Here's how the part is built. I have some questions about the finished solid (model axes, mm). A direction names the side the tool comes from. Coordinates: 2 decimals unless noted, no trailing zeros. Write each loop counter-clockwise with the first axis right and the second up, starting at its lowest first coordinate (ties: lowest second). Pieces come first, ordered by that corner, then holes. Notation, with made-up numbers: (76.5, 18) -> (93.5, 18) arc R14 cw to (93.5, 33) -> close; hole circle Ø2 at (-0.75, 37.5). An arc over 180 degrees is marked (long way). Put each result on its own line as item: value.
```python
from build123d import *

# Parameters (mm, degrees)
SKETCH1_W           = 40
SKETCH1_H           = 40
BOSS_EXTRUDE1_DEPTH = 25
SKETCH2_R           = 8.5
BOSS_EXTRUDE2_DEPTH = 9
SKETCH3_R           = 1
CUT_EXTRUDE1_DEPTH  = 10


with BuildPart() as part:
    # Sketch1 → Boss-Extrude1 (new body)
    with BuildSketch(Plane.XY):
        Rectangle(SKETCH1_W, SKETCH1_H)
    extrude(amount=BOSS_EXTRUDE1_DEPTH)

    # Sketch2 → Boss-Extrude2 (add)
    with BuildSketch(Plane.XZ.offset(20)):
        with Locations((0, 16.5)):
            Circle(SKETCH2_R)
    boss_extrude2 = extrude(amount=BOSS_EXTRUDE2_DEPTH)

    # Mirror1: Boss-Extrude2 across plane
    add(boss_extrude2.mirror(Plane(origin=(0, 0, 0), x_dir=(0, 0, 1), z_dir=(0.707106781, 0.707106781, 0))))

    # Sketch3 → Cut-Extrude1 (cut)
    with BuildSketch(Plane.XY.offset(25)):
        with Locations((-16.263455967, 16.263455967)):
            Circle(SKETCH3_R)
        with Locations((16.263455967, 16.263455967)):
            Circle(SKETCH3_R)
        with Locations((-16.263455967, -16.263455967)):
            Circle(SKETCH3_R)
        with Locations((16.263455967, -16.263455967)):
            Circle(SKETCH3_R)
    extrude(amount=-CUT_EXTRUDE1_DEPTH, mode=Mode.SUBTRACT)


solid = part.part
```
Item 1: Which directions (+Z, -Z, +X, -X, +Y, -Y) give clear straight access to the entire face, cutting with the end or side of a thin tool? Please do faces 4 (the flat face through (0, 0, 0)), 5 (the flat face through (-16, 16, 15)), 6 (the cylindrical face through (24.44, 1.84, 8.2)), 7 (the cylindrical face through (-1.84, -24.44, 8.2)), 8 (the flat face through (0, 0, 25)).
Output:
face 4: -Z, +X, -X, +Y, -Y
face 5: +Z
face 6: +X
face 7: -Y
face 8: +Z, +X, -X, +Y, -Y
Item 2: Imagine slicing it at B-B on y = -10. Write out the boundary of the cut face in (x, z).
Output:
outline: (-20, 0) -> (20, 0) -> (20, 25) -> (-20, 25) -> close
Item 3: If we mould it in two halves opening along Y, with no side actions, what happens to faces 1 (the flat face through (-20, 0, 12)), 2 (the cylindrical face through (16.133, -15.272, 20.07)), 3 (the flat face through (0, 20, 12))? For each: released by +Y, released by -Y, zero draft, split by the parting line, or undercut.
Output:
face 1: zero draft
face 2: undercut
face 3: released by +Y
Item 4: Imagine slicing it at C-C on z = 11. Write out the boundary of the cut face in (x, y), then the cut area to 3 significant figures.
Output:
outline: (-20, -20) -> (-6.48, -20) -> (-6.48, -29) -> (6.48, -29) -> (6.48, -20) -> (20, -20) -> (20, -6.48) -> (29, -6.48) -> (29, 6.48) -> (20, 6.48) -> (20, 20) -> (-20, 20) -> close
area: 1,830 mm²
Item 5: Please list where these lines run through material, in increasing order: line 1 along Y through (x, z) = (17, 22.5); line 2 along X through (y, z) = (16, 18.25); line 3 along X through (y, z) = (17.5, 11.5). Write a range as from..to.
Output:
line 1: y = -20..-16.94, -15.59..15.59, 16.94..20
line 2: x = -20..-17.23, -15.3..15.3, 17.23..20
line 3: x = -20..20
Item 6: Imagine slicing it at A-A on z = 16.5. Write out the boundary of the cut face in (x, y).
Output:
outline: (-20, -20) -> (-8.5, -20) -> (-8.5, -29) -> (8.5, -29) -> (8.5, -20) -> (20, -20) -> (20, -8.5) -> (29, -8.5) -> (29, 8.5) -> (20, 8.5) -> (20, 20) -> (-20, 20) -> close; hole circle Ø2 at (-16.26, -16.26); hole circle Ø2 at (-16.26, 16.26); hole circle Ø2 at (16.26, -16.26); hole circle Ø2 at (16.26, 16.26)
Item 7: For P1, Ø1.2, axis at x = 16.26, y = 16.26, coming from the +Z side; P2, Ø3, axis at x = 22.5, z = 17, coming from the -Y side; P3, Ø1, axis at y = -5.5, z = 5, coming from the +X side, each with a flat end and sliding along its axis, tell me the tip position at first contact or that it passes through.
Output:
P1: stops at z = 15
P2: stops at y = -8.5
P3: stops at x = 20
